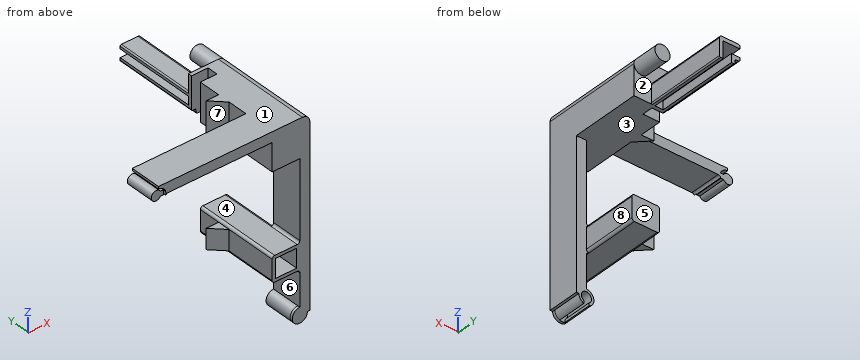
from build123d import *
from build123d.topology import SkipClean

# Parameters (mm, degrees)
SKETCH1_W                 = 30
SKETCH1_H                 = 30
BOSS_EXTRUDE1_DEPTH       = 80
SKETCH2_R                 = 6
BOSS_EXTRUDE2_DEPTH       = 20
CUT_EXTRUDE1_DEPTH        = 83.764726786
BOSS_EXTRUDE3_DEPTH       = 65
BOSS_EXTRUDE5_DEPTH       = 2
BOSS_EXTRUDE6_DEPTH       = 23
BOSS_EXTRUDE7_DEPTH       = 25
FILLET1_R                 = 2
SKETCH11_R                = 6.055782361
CUT_EXTRUDE2_DEPTH        = 2.125
CUT_EXTRUDE4_DEPTH        = 238.593079129
CUT_EXTRUDE4_DEPTH_BACK   = 238.593079129
SKETCH13_W                = 13.25
SKETCH13_H                = 8.5
FILLET2_R                 = 2
CUT_EXTRUDE6_REACH        = 195.534
SKETCH16_W                = 3.75
SKETCH16_H                = 3.75
FILLET4_R                 = 1
BOSS_EXTRUDE8_REACH       = 230.211
SKETCH17_W                = 22
SKETCH17_H                = 20
SKETCH18_W                = 17
SKETCH18_H                = 15
CUT_EXTRUDE7_DEPTH        = 66
FILLET5_R                 = 2
FILLET6_R                 = 2
CHAMFER1_SIZE             = 7
BOSS_EXTRUDE9_DEPTH       = 30
BOSS_EXTRUDE10_DEPTH      = 8
BOSS_EXTRUDE10_DEPTH_BACK = 8


with BuildPart() as part:
    # Sketch1 → Boss-Extrude1 (new body)
    with BuildSketch(Plane(origin=(0, 0, 0), x_dir=(1, 0, 0), z_dir=(0, 1, 0))):
        Rectangle(SKETCH1_W, SKETCH1_H)
    extrude(amount=BOSS_EXTRUDE1_DEPTH)

    # Sketch2 → Boss-Extrude2 (add)
    with BuildSketch(Plane(origin=(0, 80, 0), x_dir=(1, 0, 0), z_dir=(0, 1, 0))):
        with Locations(Location((9, -9, 0), (0, 0, 270))):
            Circle(SKETCH2_R)
    extrude(amount=BOSS_EXTRUDE2_DEPTH)

    # Sketch3 → Cut-Extrude1 (cut, through all)
    with BuildSketch(Plane(origin=(0, 80, 0), x_dir=(1, 0, 0), z_dir=(0, 1, 0))):
        with BuildLine():
            Line((9, -15), (15, -15))
            Line((15, -15), (15, -9))
            ThreePointArc((15, -9), (13.242640687, -13.242640687), (9, -15))
        make_face()
    extrude(amount=-CUT_EXTRUDE1_DEPTH, mode=Mode.SUBTRACT)

    # Sketch4 → Boss-Extrude3 (add)
    with BuildSketch(Plane(origin=(0, 80, 0), x_dir=(1, 0, 0), z_dir=(0, 1, 0))):
        Polygon((-11.25, 1.75), (-1.75, 1.75), (-1.75, 11.25), (-1.75, 15), (1.25, 15), (1.25, 11.25), (1.25, -1.25), (-11.25, -1.25), (-15, -1.25), (-15, 1.75), align=None)
        Polygon((-11.25, 8.25), (-8.25, 8.25), (-8.25, 11.25), (-8.25, 15), (-11.25, 15), (-11.25, 11.25), (-15, 11.25), (-15, 8.25), align=None)
    extrude(amount=BOSS_EXTRUDE3_DEPTH)

    # Sketch6 → Boss-Extrude5 (add)
    with BuildSketch(Plane.XZ):
        with BuildLine():
            Line((15, -15), (7, -15))
            Line((7, -15), (7, -126.175))
            ThreePointArc((7, -126.175), (2.757359313, -136.417640687), (13, -132.175))
            Line((13, -132.175), (15, -132.175))
            Line((15, -132.175), (15, -15))
        make_face()
    extrude(amount=-BOSS_EXTRUDE5_DEPTH)

    # Sketch7 → Boss-Extrude6 (add)
    with SkipClean():  # the faces are left unmerged after this step: merging them gives an invalid solid
        with BuildSketch(Plane(origin=(0, 2, 0), x_dir=(1, 0, 0), z_dir=(0, 1, 0))):
            with BuildLine():
                Line((9, 137.831854249), (9, 135.639101615))
                ThreePointArc((9, 135.639101615), (7, 128.175), (5, 135.639101615))
                Line((5, 135.639101615), (5, 137.831854249))
                ThreePointArc((5, 137.831854249), (1.086408642, 131.160388128), (7, 126.175))
                Line((7, 126.175), (7, 15))
                Line((7, 15), (15, 15))
                Line((15, 15), (15, 132.175))
                Line((15, 132.175), (13, 132.175))
                ThreePointArc((13, 132.175), (11.898979486, 135.639101615), (9, 137.831854249))
            make_face()
        extrude(amount=BOSS_EXTRUDE6_DEPTH)

    # Sketch9 → Boss-Extrude7 (add)
    with SkipClean():  # the faces are left unmerged after this step: merging them gives an invalid solid
        with BuildSketch(Plane.XZ):
            with BuildLine():
                Line((-15, 15), (-15, 7))
                Line((-15, 7), (-99.5, 7))
                ThreePointArc((-99.5, 7), (-99.577697751, 6.037536458), (-99.80877869, 5.1))
                Line((-99.80877869, 5.1), (-102.122778509, 5.1))
                ThreePointArc((-102.122778509, 5.1), (-109.375, 7), (-102.122778509, 8.9))
                Line((-102.122778509, 8.9), (-99.625, 8.9))
                ThreePointArc((-99.625, 8.9), (-101.816885554, 11.955834237), (-105.375001601, 13.173329766))
                Line((-105.375001601, 13.173329766), (-105.375001601, 15))
                Line((-105.375001601, 15), (-15, 15))
            make_face()
        extrude(amount=-BOSS_EXTRUDE7_DEPTH)

    # Fillet1
    fillet1_edges = [part.edges().sort_by_distance(p)[0] for p in [
        (-99.5, 12.5, 7),
    ]]
    fillet(fillet1_edges, radius=FILLET1_R)

    # Sketch11 → Cut-Extrude2 (cut)
    with SkipClean():  # the faces are left unmerged after this step: merging them gives an invalid solid
        with BuildSketch(Plane.XZ):
            with Locations((-105.5, 7)):
                Circle(SKETCH11_R)
        extrude(amount=-CUT_EXTRUDE2_DEPTH, mode=Mode.SUBTRACT)

    # Sketch13 → Cut-Extrude4 (cut, two sides: drawn at the far end of the back side and taken through both)
    with SkipClean():  # the faces are left unmerged after this step: merging them gives an invalid solid
        with BuildSketch(Plane.XY.offset(15).offset(-CUT_EXTRUDE4_DEPTH_BACK)):
            with Locations((-8.375, 72.75)):
                Rectangle(SKETCH13_W, SKETCH13_H)
        extrude(amount=CUT_EXTRUDE4_DEPTH + CUT_EXTRUDE4_DEPTH_BACK, mode=Mode.SUBTRACT)

    # Fillet2
    fillet2_edges = [part.edges().sort_by_distance(p)[0] for p in [
        (1.25, 112.5, 1.25),
    ]]
    fillet(fillet2_edges, radius=FILLET2_R)

    # Sketch16 → Cut-Extrude6 (cut, up to next)
    with BuildSketch(Plane(origin=(0, 80, 0), x_dir=(1, 0, 0), z_dir=(0, 1, 0)), mode=Mode.PRIVATE) as cut_extrude6_sk1:
        with Locations((-13.125, 13.125)):
            Rectangle(SKETCH16_W, SKETCH16_H)
    cut_extrude6_tool1 = extrude(cut_extrude6_sk1.sketch, amount=-CUT_EXTRUDE6_REACH, mode=Mode.PRIVATE) & part.part
    add(cut_extrude6_tool1.solids().sort_by_distance((-13.125, 80, -13.125))[0], mode=Mode.SUBTRACT)

    # Fillet4
    fillet4_edges = [part.edges().sort_by_distance(p)[0] for p in [
        (-11.25, 112.5, -11.25),
        (-15, 112.5, -11.25),
        (-11.25, 112.5, -15),
        (-15, 112.5, 1.25),
        (1.25, 112.5, -15),
    ]]
    fillet(fillet4_edges, radius=FILLET4_R)

    # Boss-Extrude8: up to this face of the body (flat: up to its plane)
    boss_extrude8_end = Plane(part.part.faces().sort_by_distance((-8.375, 68.5, 0))[0])
    # Sketch17 → Boss-Extrude8 (add, up to the picked face)
    with BuildSketch(Plane.XZ, mode=Mode.PRIVATE) as boss_extrude8_sk1:
        with Locations((-4, -88.38125)):
            Rectangle(SKETCH17_W, SKETCH17_H)
    boss_extrude8_tool1 = split(extrude(boss_extrude8_sk1.sketch, amount=-BOSS_EXTRUDE8_REACH, mode=Mode.PRIVATE), bisect_by=boss_extrude8_end, keep=Keep.BOTH, mode=Mode.PRIVATE)
    add(boss_extrude8_tool1.solids().sort_by(Axis((-4, 0, -88.38125), (0, 1, 0)))[0])

    # Sketch18 → Cut-Extrude7 (cut)
    with SkipClean():  # the faces are left unmerged after this step: merging them gives an invalid solid
        with BuildSketch(Plane.XZ):
            with Locations((-4, -88.38125)):
                Rectangle(SKETCH18_W, SKETCH18_H)
        extrude(amount=-CUT_EXTRUDE7_DEPTH, mode=Mode.SUBTRACT)

    # Fillet5
    fillet5_edges = [part.edges().sort_by_distance(p)[0] for p in [
        (7, 13.5, -78.38125),
        (7, 13.5, -98.38125),
        (-15, 34.25, -98.38125),
        (-15, 34.25, -78.38125),
    ]]
    fillet(fillet5_edges, radius=FILLET5_R)

    # Fillet6
    fillet6_edges = [part.edges().sort_by_distance(p)[0] for p in [
        (7, 46.75, -78.38125),
        (7, 46.75, -98.38125),
    ]]
    fillet(fillet6_edges, radius=FILLET6_R)

    # Chamfer1
    chamfer1_edges = [part.edges().sort_by_distance(p)[0] for p in [
        (-12.5, 66, -88.38125),
        (-4, 66, -80.88125),
        (4.5, 66, -88.38125),
        (-4, 66, -95.88125),
    ]]
    chamfer(chamfer1_edges, length=CHAMFER1_SIZE)

    # Sketch19 → Boss-Extrude9 (add)
    with SkipClean():  # the faces are left unmerged after this step: merging them gives an invalid solid
        with BuildSketch(Plane.XY.offset(15)):
            Polygon((-15, 51), (-25, 51), (-15, 41), align=None)
        extrude(amount=-BOSS_EXTRUDE9_DEPTH)

    # Sketch20 → Boss-Extrude10 (add, two sides: drawn at the far end of the back side and taken through both)
    with SkipClean():  # the faces are left unmerged after this step: merging them gives an invalid solid
        with BuildSketch(Plane(origin=(0, 0, -88.38125), x_dir=(-1, 0, 0), z_dir=(0, 0, -1)).offset(-BOSS_EXTRUDE10_DEPTH_BACK)):
            Polygon((25, 51), (15, 51), (15, 41), align=None)
        extrude(amount=BOSS_EXTRUDE10_DEPTH + BOSS_EXTRUDE10_DEPTH_BACK)


solid = part.part
Geometry: final body of the model. Coordinates: model frame, mm. Face numbers are marked on the shaded views. A direction names the side the tool comes from. Give positions to 0.01 mm unless a question says otherwise; leave off trailing zeros. Loops run counter-clockwise (first coordinate to the right, second up) from the corner with the lowest first, then second, coordinate; pieces in that order, holes last. Notation, with made-up numbers: (-35.75, 47) -> (-0.75, 47) arc R16 ccw to (-0.75, 59) -> close; hole circle Ø4 at (-3.5, -20). An arc over 180 degrees is marked (long way). Put each result on its own line as item: value.
1. Ray query, line 1 along Z through (x, y) = (3.5, 10.5); line 2 along X through (y, z) = (136.5, -1); line 3 along Y through (x, z) = (9, -80). Return the intervals inside material, ascending. Write a range as [from, to].
Taken from the geometry:
line 1: z = [-137.05, -134.11], [-130.24, -127.3], [-98.38, -95.88], [-80.88, -78.38], [-15, 15]
line 2: x = [-15, 1.25]
line 3: y = [0, 25]
2. Cut plane D-D (z = -92). Return the cut outline in (x, y), plus the area to 3 significant figures.
Taken from the geometry:
outline: (-25, 51) -> (-15, 41) -> (-15, 0) -> (-12.5, 0) -> (-12.5, 59) -> (-8.62, 62.88) -> (0.62, 62.88) -> (4.5, 59) -> (4.5, 0) -> (15, 0) -> (15, 25) -> (7, 25) -> (7, 68.5) -> (-15, 68.5) -> (-15, 51) -> close
area: 703 mm2
3. Pull-direction query (Z, two-part tool) for the marked faces 1, 2, 3 and 4; classes: released by +Z, released by -Z, zero draft, split by the parting line, or undercut.
Taken from the geometry:
face 1: released by +Z
face 2: zero draft
face 3: undercut
face 4: undercut
4. Set-up query: the marked faces 5, 6, 7 and 8. Return all of +Z, -Z, +X, -X, +Y, -Y with unobstructed straight access to the full face (end or side cutting, diameter ignored); none if empty.
Taken from the geometry:
face 5: -Z, +X, -X, +Y
face 6: -X, +Y, -Y
face 7: +Z, -Z, -X
face 8: -Z, +X, +Y
5. Cut plane B-B (y = 107). Return the cut outline in (x, z), plus the area to 3 significant figures.
Taken from the geometry:
outline: (-15, -10.25) arc R1 ccw to (-14, -11.25) -> (-12.25, -11.25) arc R1 cw to (-11.25, -12.25) -> (-11.25, -14) arc R1 ccw to (-10.25, -15) -> (-8.25, -15) -> (-8.25, -8.25) -> (-15, -8.25) -> close; (-15, -1.75) -> (-1.75, -1.75) -> (-1.75, -15) -> (0.25, -15) arc R1 ccw to (1.25, -14) -> (1.25, -0.75) arc R2 ccw to (-0.75, 1.25) -> (-14, 1.25) arc R1 ccw to (-15, 0.25) -> close
area: 118 mm2
6. Cut plane A-A (y = 48). Return the cut outline in (x, z).
Taken from the geometry:
outline: (-22, -96.38) -> (-15, -96.38) arc R2 ccw to (-13, -98.38) -> (5, -98.38) arc R2 ccw to (7, -96.38) -> (7, -80.38) arc R2 ccw to (5, -78.38) -> (-13, -78.38) arc R2 ccw to (-15, -80.38) -> (-22, -80.38) -> close; (-22, -15) -> (15, -15) -> (15, 9) arc R6 ccw to (9, 15) -> (-22, 15) -> close; hole (-12.5, -95.88) -> (4.5, -95.88) -> (4.5, -80.88) -> (-12.5, -80.88) -> close
7. Pin query (flat end, axial travel): P1, Ø2.5, axis at x = 8.5, z = -132.5, coming from the +Y side; P2, Ø14.5, axis at x = -8, y = 106, coming from the +Z side; P3, Ø6, axis at x = -5, y = 111.5, coming from the -Z side; P4, Ø14.5, axis at x = -9, z = -6.5, coming from the +Y side. Return the tip coordinate at first contact, or that it passes through.
Taken from the geometry:
P1: stops at y = 2
P2: stops at z = 1.25
P3: stops at z = -1.75
P4: stops at y = 145
